Build history of the part. All positions in model axes, mm. Face numbers are marked on the shaded views. A direction names the side the tool comes from. Round coordinates to 2 decimals unless told otherwise and drop trailing zeros. Write each loop counter-clockwise with the first axis right and the second up, starting at its lowest first coordinate (ties: lowest second). Pieces come first, ordered by that corner, then holes. Notation, with made-up numbers: M 54,-13 L 83,-13 A23 cw 83,4 Z; hole C 21,63 d5. An arc over 180 degrees is marked long. Write item = value, one per line.
from build123d import *

# Parameters (mm, degrees)
F0_W     = 72.6709449252
F0_H     = 47
F0_R     = 1
F0_W_2   = 58.4303468724
F0_H_2   = 33.0635516279
F1_DEPTH = 3
F2_W     = 3
F2_H     = 47
F3_DEPTH = 16
F4_R     = 3
F5_DEPTH = 47
F6_R     = 2
F7_DEPTH = 59
F8_W     = 58.4303468724
F8_H     = 26.9109723158
F9_DEPTH = 25


with BuildPart() as f1:
    # F0 (on Top) → F1 (new body)
    with BuildSketch(Plane.XY):
        with Locations((-6.0011862931, 6.6216193669)):
            Rectangle(F0_W, F0_H)
        with Locations((-38.4287770241, -13.4855430331)):
            Circle(F0_R, mode=Mode.SUBTRACT)
        with Locations((-6.0011862931, 6.6216193669)):
            Rectangle(F0_W_2, F0_H_2, mode=Mode.SUBTRACT)
        with Locations((26.3990384156, -13.4553477725)):
            Circle(F0_R, mode=Mode.SUBTRACT)
        with Locations((-38.4287770241, 27.9226825441)):
            Circle(F0_R, mode=Mode.SUBTRACT)
        with Locations((26.426404438, 26.7287817669)):
            Circle(F0_R, mode=Mode.SUBTRACT)
    extrude(amount=F1_DEPTH)

    # F2 (on face) → F3 (join)
    with BuildSketch(Plane.XY.offset(3)):
        with Locations((31.8342861695, 6.6216193669)):
            Rectangle(F2_W, F2_H)
        with Locations((-43.8366587557, 6.6216193669)):
            Rectangle(F2_W, F2_H)
    extrude(amount=-F3_DEPTH)

    # F4 (on face) → F5 (join)
    with BuildSketch(Plane(origin=(0, 30.1216193669, 0), x_dir=(-1, 0, 0), z_dir=(0, 1, 0))):
        with Locations((-19.05452002, -2.8200918249)):
            Circle(F4_R)
        with Locations((30.9695991276, -1.7886548301)):
            Circle(F4_R)
    extrude(amount=-F5_DEPTH)

    # F6 (on face) → F7 (cut)
    with BuildSketch(Plane(origin=(0, 30.1216193669, 0), x_dir=(-1, 0, 0), z_dir=(0, 1, 0))):
        with Locations((30.9695991276, -1.7886548301)):
            Circle(F6_R)
        with Locations((-19.05452002, -2.8200918249)):
            Circle(F6_R)
    extrude(amount=-F7_DEPTH, mode=Mode.SUBTRACT)

    # F8 (on face) → F9 (cut)
    with BuildSketch(Plane.XY.offset(3)):
        with Locations((-6.0011862931, 7.0818343665)):
            Rectangle(F8_W, F8_H)
    extrude(amount=-F9_DEPTH, mode=Mode.SUBTRACT)


solid = f1.part
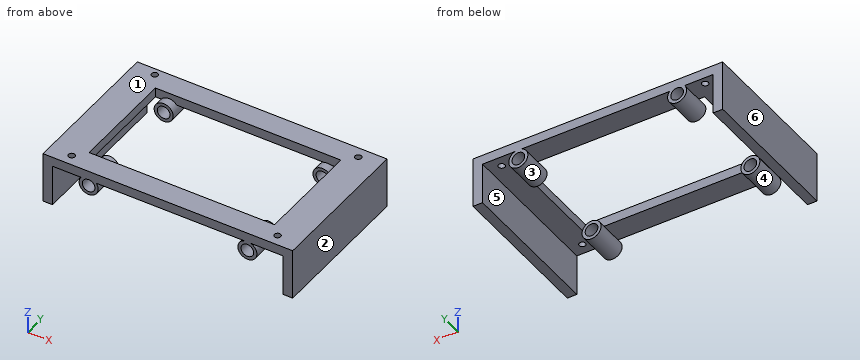
1. Band-saw the part on A-A (y = 2). List the corners of the cut face in (x, z), plus the area to 3 significant figures.
Responses:
outline = M -45.34,-13 L -42.34,-13 L -42.34,0 L -35.22,0 L -35.22,3 L -45.34,3 Z; M 23.21,0 L 30.33,0 L 30.33,-13 L 33.33,-13 L 33.33,3 L 23.21,3 Z
area = 139 mm²
2. Band-saw the part on B-B (z = -9.75). List the corners of the cut face in (x, y).
Responses:
outline = M -45.34,-16.88 L -42.34,-16.88 L -42.34,30.12 L -45.34,30.12 Z; M 30.33,-16.88 L 33.33,-16.88 L 33.33,30.12 L 30.33,30.12 Z
3. Tool access for the marked faces 5 and 6: list every direction of +Z, -Z, +X, -X, +Y, -Y with a clear straight run to the whole face (end or side of a thin tool).
Responses:
face_5 = -Z, +Y, -Y
face_6 = +Z, -Z, -X, +Y, -Y
4. Flat gauge pins, fed straight in: pin 1 (1.5 mm diameter, centred on x = -17.5, z = -0.5, fed in from +Y); pin 2 (2.5 mm diameter, centred on x = -38.43, y = 27.92, fed in from -Z); pin 3 (1.6 mm diameter, centred on x = 26.4, y = -13.46, fed in from +Z). Where does each tip first touch, or does it go through?
Responses:
pin_1 = 30.12
pin_2 = 0
pin_3 = through
5. Band-saw the part on D-D (x = -30). List the corners of the cut face in (y, z).
Responses:
outline = M -16.88,-4.63 L -6.37,-4.63 L -6.37,-3.54 L -16.88,-3.54 Z; M -16.88,-0.04 L -6.37,-0.04 L -6.37,1.05 L -9.91,1.05 L -9.91,3 L -16.88,3 Z; M 20.54,-4.63 L 30.12,-4.63 L 30.12,-3.54 L 20.54,-3.54 Z; M 20.54,-0.04 L 30.12,-0.04 L 30.12,3 L 23.15,3 L 23.15,1.05 L 20.54,1.05 Z
6. Probe probe 1 along X at (y, z) = (19, -11); probe 2 along Y at (x, z) = (10.5, 2.25); probe 3 along X at (y, z) = (15, 2.25). List the from-to ranges inside material, lowest first.
Responses:
probe_1 = -45.34 to -42.34, 30.33 to 33.33
probe_2 = -16.88 to -9.91, 23.15 to 30.12
probe_3 = -45.34 to -35.22, 23.21 to 33.33
7. Mould opens along Z. For the marked faces 1, 2, 3 and 4 say: pulls with the +Z half, pulls with the -Z half, needs draft (parallel to the pull), parting line crosses it, or undercut.
Responses:
face_1 = pulls with the +Z half
face_2 = needs draft
face_3 = undercut
face_4 = undercut
8. Band-saw the part on C-C (x = -18.5). List the corners of the cut face in (y, z), plus the area to 3 significant figures.
Responses:
outline = M -16.88,0 L -9.91,0 L -9.91,3 L -16.88,3 Z; M 23.15,0 L 30.12,0 L 30.12,3 L 23.15,3 Z
area = 41.8 mm²
